Here's how the part is built. I have some questions about the finished solid (model axes, mm). A direction names the side the tool comes from. Coordinates: 2 decimals unless noted, no trailing zeros. Loops run counter-clockwise (first coordinate to the right, second up) from the corner with the lowest first, then second, coordinate; pieces in that order, holes last. Notation, with made-up numbers: (63.25, 18) -> (82.25, 18) arc R13 cw to (82.25, 29) -> close; hole circle Ø5 at (-27.5, -27). An arc over 180 degrees is marked (long way). Answer as a JSON object with one key per item and string values. Group by question number.
Q1. I need wall thicknesses on line 1 (Y direction, x = 10, z = 5); line 2 (Z direction, x = 25.5, y = 15); line 3 (Y direction, x = -2, z = 4.5). Which ranges of each line are inside material? Lowest first, please.
Q2. I'm going to push flat-ended pins straight in: pin 1 (6 mm diameter, centred on y = 7, z = 8, fed in from +X); pin 2 (3 mm diameter, centred on y = -6.5, z = 1.5, fed in from -X); pin 3 (6 mm diameter, centred on x = 14.5, y = -8.5, fed in from +Z); pin 4 (5 mm diameter, centred on y = 13.5, z = 7, fed in from -X). Where does each tip first touch, or does it pass through?
Q3. On a 3-axis mill with a long thin cutter (end or side, diameter ignored), from which of +Z, -Z, +X, -X, +Y, -Y can I reach the whole of each face in a straight line? I mean faces 1 (the flat face through (0, -18, 1)), 2 (the cylindrical face through (-15, 0, 6)), 3 (the flat face through (-1, -8, 3)), 4 (the flat face through (0, -5, 6)). Say none if no direction works.
Q4. I want a section at A-A on z = 7. Write out the boundary of the cut face in (x, y), then the cut area to 3 significant figures.
Q5. I want a section at C-C on z = 2.25. Write out the boundary of the cut face in (x, y), then the cut area to 3 significant figures.
Q6. I want a section at B-B on y = -14. Write out the boundary of the cut face in (x, z), then the cut area to 3 significant figures.
Q7. I want a section at D-D on x = 30. Write out the boundary of the cut face in (y, z), then the cut area to 3 significant figures.
Q8. Thinking about a two-plate mould opening in X: for faces 5 (the flat face through (0, 5, 6)), 6 (the cylindrical face through (9.63, -1.66, 5.64)), 7 (the cylindrical face through (15, 0, 6)), which applies, released by +X, released by -X, zero draft, split by the parting line, or undercut?
```python
from build123d import *

# Parameters (mm, degrees)
EXTRUDE_1_DEPTH = 3
SKETCH_1_3_R    = 3.2
SKETCH_1_3_R_2  = 1.7
EXTRUDE_2_DEPTH = 10
CHAMFER_1_SIZE  = 1.4


with BuildPart() as part:
    # Sketch 1 → Extrude 1 (new body)
    with BuildSketch(Plane.XY):
        with BuildLine():
            Line((-18, -18), (18, -18))
            ThreePointArc((18, -18), (36, 0), (18, 18))
            Line((18, 18), (-18, 18))
            ThreePointArc((-18, 18), (-36, 0), (-18, -18))
        make_face()
        with BuildLine():
            ThreePointArc((10, -5), (15, 0), (10, 5))
            Line((10, 5), (-10, 5))
            ThreePointArc((-10, 5), (-15, 0), (-10, -5))
            Line((-10, -5), (10, -5))
        make_face(mode=Mode.SUBTRACT)
    extrude(amount=EXTRUDE_1_DEPTH)

    # Sketch 1_3 → Extrude 2 (add)
    # profile 1 of 3: a face of its own
    with BuildSketch(Plane.XY):
        with BuildLine():
            Line((-10, -5), (10, -5))
            ThreePointArc((10, -5), (15, 0), (10, 5))
            Line((10, 5), (-10, 5))
            ThreePointArc((-10, 5), (-15, 0), (-10, -5))
        make_face()
        with Locations((10, 0)):
            Circle(SKETCH_1_3_R, mode=Mode.SUBTRACT)
        with Locations((-10, 0)):
            Circle(SKETCH_1_3_R, mode=Mode.SUBTRACT)
    # profile 2 of 3: a face of its own
    with BuildSketch(Plane.XY):
        with Locations((-10, 0)):
            Circle(SKETCH_1_3_R)
        with Locations((-10, 0)):
            Circle(SKETCH_1_3_R_2, mode=Mode.SUBTRACT)
    # profile 3 of 3: a face of its own
    with BuildSketch(Plane.XY):
        with Locations((10, 0)):
            Circle(SKETCH_1_3_R)
        with Locations((10, 0)):
            Circle(SKETCH_1_3_R_2, mode=Mode.SUBTRACT)
    extrude(amount=EXTRUDE_2_DEPTH)

    # Chamfer 1
    chamfer_1_edges = [part.edges().sort_by_distance(p)[0] for p in [
        (-11.7, 0, 0),
        (8.3, 0, 0),
    ]]
    chamfer(chamfer_1_edges, length=CHAMFER_1_SIZE)


solid = part.part
```
Result set:
{
 "1": {"line 1": "y = -5 to -1.7, 1.7 to 5", "line 2": "z = 0 to 3", "line 3": "y = -5 to 5"},
 "2": {"pin 1": "stops at x = 13", "pin 2": "stops at x = -35.29", "pin 3": "stops at z = 3", "pin 4": "passes through"},
 "3": {"face 1": "+Z, -Z, +X, -X, -Y", "face 2": "+Z, -X", "face 3": "+Z", "face 4": "+Z, +X, -X, -Y"},
 "4": {"outline": "(-10, -5) -> (10, -5) arc R5 ccw to (10, 5) -> (-10, 5) arc R5 ccw to start; hole circle Ø3.4 at (-10, 0); hole circle Ø3.4 at (10, 0)", "area": "260 mm²"},
 "5": {"outline": "(-18, -18) -> (18, -18) arc R18 ccw to (18, 18) -> (-18, 18) arc R18 ccw to start; hole circle Ø3.4 at (-10, 0); hole circle Ø3.4 at (10, 0)", "area": "2,300 mm²"},
 "6": {"outline": "(-29.31, 0) -> (29.31, 0) -> (29.31, 3) -> (-29.31, 3) -> close", "area": "176 mm²"},
 "7": {"outline": "(-13.42, 0) -> (13.42, 0) -> (13.42, 3) -> (-13.42, 3) -> close", "area": "80.5 mm²"},
 "8": {"face 5": "zero draft", "face 6": "undercut", "face 7": "released by +X"}
}
